Geometry: final body of the model. Coordinates: model frame, mm. A direction names the side the tool comes from. Coordinates: 2 decimals unless noted, no trailing zeros. Write each loop counter-clockwise with the first axis right and the second up, starting at its lowest first coordinate (ties: lowest second). Pieces come first, ordered by that corner, then holes. Notation, with made-up numbers: (47, -16.75) - (70, -16.75) arc R9 cw to (70, -6.75) - close; hole circle Ø8 at (67.25, 27.5). An arc over 180 degrees is marked (long way). Answer as a JSON object with one key per item and string values. Group by question number.
Item 1: Line query: line 1 along Y through (x, z) = (92, 1.6); line 2 along Y through (x, z) = (103.25, 1.4); line 3 along X through (y, z) = (67, 1.4). Output: solid intervals per line, ascending. Write a range as from..to.
Item 2: Set-up query: faces 1 (the flat face through (69, 68, 3)), 2 (the cylindrical face through (86.05, 26.96, 1.48)). Return all of +Z, -Z, +X, -X, +Y, -Y with unobstructed straight access to the full face (end or side cutting, diameter ignored); none if empty.
Item 3: Section A-A on y = 84. Return loops of the section in (x, z).
Item 4: Section B-B on z = 1.85. State how many separate pieces and enclosed holes the cut face has, and give its area (3 significant figures).
Item 5: Mould query, pull axis Y, two halves, no side actions, for faces 3 (the flat face through (69, 68, 0)), 4 (the cylindrical face through (81, 124, 2)). Classes: pulls with the +Y half, pulls with the -Y half, needs draft (parallel to the pull), parting line crosses it, or undercut.
Item 6: First-contact query: pin 1 Ø0.9 at (x, z) = (136, 1.5) entering from +Y; pin 2 Ø5 at (x, y) = (34.5, 37) entering from +Z; pin 3 Ø1.5 at (x, z) = (141.5, 2) entering from -Y; pin 4 Ø0.9 at (x, z) = (64.5, 2) entering from -Y. Flat tips, straight axial feed; report the tip coordinate or a pass-through.
Autodesk Inventor part; units mm, degrees
ref_plane "YZ Plane" through (0, 0, 0) normal (1, 0, 0) x (0, 1, 0)
ref_plane "XZ Plane" through (0, 0, 0) normal (0, 1, 0) x (-1, 0, 0)
ref_plane "XY Plane" through (0, 0, 0) normal (0, 0, 1) x (1, 0, 0)
sketch "Sketch1" plane through (0, 0, 0) normal (0, 0, 1) x (1, 0, 0)
  line L0 (0, 0) -> (140, 0)
  line L1 (140, 0) -> (140, 134)
  line L2 (140, 134) -> (0, 134)
  line L3 (0, 134) -> (0, 0)
  line L4 (30, 137) -> (45, 137)
  line L5 (45, 137) -> (45, -3)
  line L6 (45, -3) -> (30, -3)
  line L7 (30, -3) -> (30, 137)
  line L8 (100, 137) -> (110, 137)
  line L9 (110, 137) -> (110, -3)
  line L10 (110, -3) -> (100, -3)
  line L11 (100, -3) -> (100, 137)
  line L12 (-3, 124) -> (0, 124)
  line L13 (0, 124) -> (0, 114)
  line L14 (0, 114) -> (-3, 114)
  line L15 (-3, 114) -> (-3, 124)
  line L16 (-3, 20) -> (0, 20)
  line L17 (0, 20) -> (0, 10)
  line L18 (0, 10) -> (-3, 10)
  line L19 (-3, 10) -> (-3, 20)
  line L20 (-3, 72) -> (0, 72)
  line L21 (0, 72) -> (0, 62)
  line L22 (0, 62) -> (-3, 62)
  line L23 (-3, 62) -> (-3, 72)
  line L24 (140, 109) -> (143, 109)
  line L25 (143, 109) -> (143, 99)
  line L26 (143, 99) -> (140, 99)
  line L27 (140, 99) -> (140, 109)
  line L28 (140, 35) -> (143, 35)
  line L29 (143, 35) -> (143, 25)
  line L30 (143, 25) -> (140, 25)
  line L31 (140, 25) -> (140, 35)
  dimension "d0" = 140
  dimension "d1" = 134
  dimension "d2" = 140
  dimension "d3" = 3
  dimension "d4" = 15
  dimension "d5" = 10
  dimension "d6" = 140
  dimension "d7" = 3
  dimension "d8" = 30
  dimension "d9" = 30
  dimension "d10" = 10
  dimension "d12" = 3
  dimension "d13" = 10
  dimension "d14" = 3
  dimension "d15" = 3
  dimension "d16" = 10
  dimension "d17" = 10
  dimension "d103" = 10
  dimension "d104" = 42
  dimension "d208" = 3
  dimension "d213" = 3
  dimension "d214" = 10
  dimension "d215" = 25
  dimension "d216" = 3
  dimension "d217" = 10
  dimension "d218" = 25
extrude "Extrusion1" add sketch "Sketch1" along normal blind 3
sketch "Sketch2" plane through (0, 0, 3) normal (0, 0, 1) x (1, 0, 0)
  line L0 (0, 0) -> (0, 10)
  line L1 (100, 0) -> (45, 0)
  point P0 (80.25, 3.5)
  point P1 (103.25, 26.5)
  point P2 (103.25, 3.5)
  dimension "d102" = 23
  dimension "d119" = 80.25
  dimension "d122" = 3.5
  dimension "d123" = 23
hole "Hole1" at (80.25, 3.5, 3) at (103.25, 26.5, 3) at (103.25, 3.5, 3) direction (0, 0, -1) diameter 2.5 end through all
sketch "Sketch3" plane through (0, 0, 3) normal (0, 0, 1) x (1, 0, 0)
  line L0 (0, 20) -> (0, 114)
  line L1 (30, 0) -> (0, 0)
  line L2 (0, 0) -> (0, 10)
  point P0 (3.5, 78.5)
  point P1 (3.5, 55.5)
  point P2 (26.5, 78.5)
  point P3 (26.5, 55.5)
  dimension "d35" = 23
  dimension "d37" = 3.5
  dimension "d48" = 3.5
  dimension "d93" = 55.5
  dimension "d101" = 23
  dimension "d105" = 23
hole "Hole2" at (3.5, 78.5, 3) at (3.5, 55.5, 3) at (26.5, 78.5, 3) at (26.5, 55.5, 3) direction (0, 0, -1) diameter 2.5 end through all
sketch "Sketch5" plane through (0, 0, 3) normal (0, 0, 1) x (1, 0, 0)
  line L0 (0, 124) -> (0, 134)
  line L1 (0, 0) -> (0, 10)
  line L2 (0, 134) -> (30, 134)
  line L3 (30, 0) -> (0, 0)
  point P0 (15, 122)
  point P1 (15, 12)
  dimension "d56" = 15
  dimension "d57" = 15
  dimension "d89" = 12
  dimension "d90" = 12
hole "Hole3" at (15, 122, 3) at (15, 12, 3) direction (0, 0, -1) diameter 4 end through all
sketch "Sketch6" plane through (0, 0, 3) normal (0, 0, 1) x (1, 0, 0)
  circle A0 centre (15, 122) radius 2
  circle A1 centre (15, 12) radius 2
  point P0 (6, 122)
  point P1 (24, 122)
  point P2 (6, 12)
  point P3 (24, 12)
  dimension "d65" = 9
  dimension "d66" = 9
  dimension "d67" = 9
  dimension "d68" = 9
  dimension "d91" = 0
  dimension "d92" = 0
hole "Hole4" at (6, 122, 3) at (24, 122, 3) at (6, 12, 3) at (24, 12, 3) direction (0, 0, -1) diameter 3 end through all
sketch "Sketch8" plane through (0, 0, 3) normal (0, 0, 1) x (1, 0, 0)
  line L0 (45, 134) -> (100, 134)
  line L1 (140, 134) -> (140, 109)
  point P0 (92, 125.5)
  dimension "d136" = 8.5
  dimension "d226" = 48
hole "Hole5" at (92, 125.5, 3) direction (0, 0, -1) diameter 3 end through all
sketch "Sketch13" plane through (0, 0, 3) normal (0, 0, 1) x (1, 0, 0)
  circle A0 centre (3.5, 78.5) radius 1.25
  circle A1 centre (80.25, 3.5) radius 1.25
  point P0 (15, 67)
  point P1 (91.75, 15)
  dimension "d108" = 11.5
  dimension "d109" = 11.5
  dimension "d124" = 11.5
  dimension "d125" = 11.5
hole "Hole6" at (15, 67, 3) at (91.75, 15, 3) direction (0, 0, -1) diameter 22 end through all
sketch "Sketch15" plane through (0, 0, 3) normal (0, 0, 1) x (1, 0, 0)
  line L0 (100, 0) -> (45, 0)
  line L1 (45, 134) -> (100, 134)
  line L2 (81, 124) -> (81, 124)
  line L3 (84.25, 120.75) -> (84.25, 10)
  line L4 (84.25, 10) -> (81, 10)
  line L5 (77.75, 13.25) -> (77.75, 120.75)
  arc A0 (81, 124) -> (77.75, 120.75) centre (81, 120.75) ccw
  arc A1 (84.25, 120.75) -> (81, 124) centre (81, 120.75) ccw
  arc A2 (77.75, 13.25) -> (81, 10) centre (81, 13.25) ccw
  circle A3 centre (91.75, 15) radius 11
  point P0 (77.75, 124)
  point P1 (84.25, 124)
  point P2 (77.75, 10)
  dimension "d129" = 10
  dimension "d130" = 6.5
  dimension "d131" = 3.25
  dimension "d137" = 10
  dimension "d138" = 3.25
  dimension "d224" = 14
extrude "Extrusion2" cut sketch "Sketch15" against normal through all contours L3 A3 L4 A2 L5 A0 A1 | L3 L4 A3 picked at (83.7345, 18.1015)
sketch "Sketch19" plane through (0, 0, 3) normal (0, 0, 1) x (1, 0, 0)
  line L0 (140, 0) -> (110, 0)
  line L1 (110, 134) -> (140, 134)
  line L2 (133.3, 134) -> (131, 134)
  line L3 (131, 134) -> (131, 132.25)
  line L4 (131, 132.25) -> (133.3, 132.25)
  line L5 (133.3, 132.25) -> (133.3, 134)
  line L6 (133.3, 0) -> (131, 0)
  line L7 (131, 0) -> (131, 1.75)
  line L8 (131, 1.75) -> (133.3, 1.75)
  line L9 (133.3, 1.75) -> (133.3, 0)
  line L10 (140, 134) -> (140, 0)
  line L11 (0, 134) -> (9.175, 134)
  line L12 (9.175, 134) -> (9.175, 132.75)
  line L13 (7.925, 131.5) -> (0, 131.5)
  line L14 (0, 131.5) -> (0, 134)
  line L15 (0, 0) -> (9.175, 0)
  line L16 (9.175, 0) -> (9.175, 1.25)
  line L17 (7.925, 2.5) -> (0, 2.5)
  line L18 (0, 2.5) -> (0, 0)
  arc A0 (7.925, 131.5) -> (9.175, 132.75) centre (7.925, 132.75) ccw
  arc A1 (9.175, 1.25) -> (7.925, 2.5) centre (7.925, 1.25) ccw
  point P0 (9.175, 131.5)
  point P1 (9.175, 2.5)
  dimension "d166" = 2.3
  dimension "d168" = 1.75
  dimension "d173" = 1.75
  dimension "d210" = 9
  dimension "d211" = 2.3
  dimension "d212" = 9
  dimension "d219" = 9.175
  dimension "d220" = 2.5
  dimension "d221" = 9.175
  dimension "d222" = 2.5
  dimension "d223" = 1.25
extrude "Extrusion3" cut sketch "Sketch19" against normal through all
fillet "圓角4" radius 5 2 edges at (84.25, 23.0467, 1.5) (81.952, 10, 1.5)
sketch "草圖24" plane through (0, 0, 3) normal (0, 0, 1) x (1, 0, 0)
  line L0 (140, 0) -> (133.3, 0)
  line L1 (140, 99) -> (140, 35)
  point P0 (0, 0)
  point P1 (134.5, 37)
  point P2 (34.5, 37)
  point P3 (134.5, 117)
  point P4 (34.5, 117)
  dimension "d227" = 37
  dimension "d228" = 5.5
  dimension "d229" = 100
  dimension "d230" = 80
hole "孔10" at (134.5, 37, 3) at (34.5, 37, 3) at (134.5, 117, 3) at (34.5, 117, 3) direction (0, 0, -1) diameter 3 end through all
sketch "草圖25" plane through (0, 0, 3) normal (0, 0, 1) x (1, 0, 0)
  line L0 (0, 20) -> (0, 62)
  line L1 (30, 0) -> (9.175, 0)
  point P0 (0, 0)
  point P1 (9.5, 32)
  dimension "d238" = 9.5
  dimension "d239" = 32
hole "孔11" at (9.5, 32, 3) direction (0, 0, -1) diameter 3 end through all
sketch "草圖26" plane through (0, 0, 3) normal (0, 0, 1) x (1, 0, 0)
  line L0 (0, 72) -> (0, 114)
  line L1 (9.175, 134) -> (30, 134)
  line L2 (0, 108.5) -> (4.5635, 108.5)
  line L3 (8, 108.5) -> (8, 105.5)
  line L4 (4.5635, 105.5) -> (0, 105.5)
  line L5 (0, 105.5) -> (0, 108.5)
  line L6 (6.5, 110) -> (6.5, 110)
  line L7 (6.5, 104) -> (6.5, 104)
  line L8 (8, 105.5) -> (8, 108.5)
  arc A0 (8, 108.5) -> (6.5, 110) centre (6.5, 108.5) ccw
  arc A1 (6.5, 104) -> (8, 105.5) centre (6.5, 105.5) ccw
  arc A2 (5.0476, 105.125) -> (6.5, 104) centre (6.5, 105.5) ccw
  arc A3 (6.5, 110) -> (5.0476, 108.875) centre (6.5, 108.5) ccw
  arc A4 (4.5635, 108.5) -> (5.0476, 108.875) centre (4.5635, 109) ccw
  arc A5 (5.0476, 105.125) -> (4.5635, 105.5) centre (4.5635, 105) ccw
  point P0 (0, 0)
  point P1 (8, 110)
  point P2 (5, 110)
  point P3 (8, 104)
  point P4 (5, 108.5)
  point P5 (5, 105.5)
  dimension "d249" = 3
  dimension "d250" = 25.5
  dimension "d251" = 3
  dimension "d252" = 6
  dimension "d253" = 8
  dimension "d255" = 1.5
  dimension "d256" = 0.5
extrude "擠出7" cut sketch "草圖26" against normal through all
sketch "草圖27" plane through (0, 0, 3) normal (0, 0, 1) x (1, 0, 0)
  line L0 (100, 0) -> (45, 0)
  line L1 (140, 25) -> (140, 0)
  point P0 (0, 0)
  point P1 (66.25, 14)
  point P2 (59.75, 14)
  dimension "d259" = 73.75
  dimension "d260" = 14
  dimension "d261" = 6.5
hole "孔12" at (66.25, 14, 3) at (59.75, 14, 3) direction (0, 0, -1) diameter 2 end through all
sketch "草圖28" plane through (0, 0, 3) normal (0, 0, 1) x (1, 0, 0)
  circle A0 centre (66.25, 14) radius 1
  line L0 (100, 0) -> (45, 0)
  line L1 (59.75, 6) -> (66.75, 6)
  line L2 (67.75, 5) -> (67.75, 0)
  line L3 (67.75, 0) -> (58.75, 0)
  line L4 (58.75, 0) -> (58.75, 5)
  arc A1 (59.75, 6) -> (58.75, 5) centre (59.75, 5) ccw
  arc A2 (67.75, 5) -> (66.75, 6) centre (66.75, 5) ccw
  point P0 (0, 0)
  point P1 (58.75, 6)
  point P2 (67.75, 6)
  dimension "d269" = 6
  dimension "d271" = 9
  dimension "d272" = 1.5
  dimension "d273" = 1
extrude "擠出8" cut sketch "草圖28" against normal through all contours L0 L4 A1 L1 A2 L2
properties part number "plastic_part_04"
Checks:
{
 "1": {"line 1": "0..4, 26..124, 127..134", "line 2": "-3..2.25, 4.75..25.25, 27.75..137", "line 3": "-3..4, 26..77.75, 84.25..140"},
 "2": {"face 1": "+Z, +X, -X, +Y, -Y", "face 2": "+Z, -Z"},
 "3": {"outline": "(0, 0) - (77.75, 0) - (77.75, 3) - (0, 3) - close; (84.25, 0) - (140, 0) - (140, 3) - (84.25, 3) - close"},
 "4": {"separate pieces": "1", "enclosed holes": "23", "area": "17,300 mm^2"},
 "5": {"face 3": "needs draft", "face 4": "undercut"},
 "6": {"pin 1": "y = 134", "pin 2": "z = 3", "pin 3": "y = 25", "pin 4": "y = 6"}
}
